Geometry check sheet. Reference: the model listing, model coordinates, mm. Coordinates: 2 decimals unless noted, no trailing zeros. Order: outer loops, then holes, each group sorted by start corner. A loop starts at its lowest first (then second) coordinate and runs counter-clockwise, first axis right, second up. Notation, with made-up numbers: (-23, -9) - (28, -9) arc R14 ccw to (28, 8) - close; hole circle Ø11 at (52.5, 81.5). An arc over 180 degrees is marked (long way). Use CSV: the item, a comma, the result in double quotes. Start each with the question number.
1) Sectioned sample at B-B, the plane z = -54. Record the cut outline in (x, y), and give its area (3 significant figures).
2) Depth check by flat-ended pin: P1, Ø1.2, axis at y = 0.5, z = -62.5, coming from the +X side; P2, Ø2.5, axis at x = 70, z = -39, coming from the -Y side; P3, Ø1.2, axis at y = 1, z = -60.5, coming from the -X side; P4, Ø1.5, axis at y = 1.5, z = -27.5, coming from the -X side. Enter the tip coordinate at first touch or a pass-through.
3) Sectioned sample at D-D, the plane y = 0.1. Count the separate pieces of the cut face and the enclosed holes in it, and give its area (3 significant figures).
4) Thickness scan on probe 1 along Z at (x, y) = (-16, -1.3); probe 2 along X at (y, z) = (0.35, -24.5); probe 3 along X at (y, z) = (0.5, -48). Record the ranges inside material, lowest first. Write a range as [from, to].
5) Sectioned sample at C-C, the plane x = 1. Record the cut outline in (y, z).
6) Sectioned sample at A-A, the plane x = 28. Record the cut outline in (y, z), and give its area (3 significant figures).
from build123d import *

# Parameters (mm, degrees)
F1_DEPTH = 2
F2_SIZE  = 5
F3_R     = 5
F4_R     = 1.5
F5_DEPTH = 4.001
F6_R     = 0.5
F8_DEPTH = 4.001


with BuildPart() as f1:
    # F0 (on Front) → F1 (new body, symmetric)
    with BuildSketch(Plane.XZ):
        with BuildLine():
            Line((94.041232037, 0), (-94.041232037, 0))
            ThreePointArc((-94.041232037, 0), (-97.8714542526, -1.7860619516), (-98.9652708021, -5.8682408883))
            Line((-98.9652708021, -5.8682408883), (-86.9750361139, -73.8682408883))
            ThreePointArc((-86.9750361139, -73.8682408883), (-85.2649353973, -76.8302222156), (-82.0509973489, -78))
            Line((-82.0509973489, -78), (-74, -78))
            Line((-74, -78), (-74, -39))
            Line((-74, -39), (-70, -39))
            Line((-70, -39), (-70, -78))
            Line((-70, -78), (70, -78))
            Line((70, -78), (70, -39))
            Line((70, -39), (74, -39))
            Line((74, -39), (74, -78))
            Line((74, -78), (82.0509973489, -78))
            ThreePointArc((82.0509973489, -78), (85.2649353973, -76.8302222156), (86.9750361139, -73.8682408883))
            Line((86.9750361139, -73.8682408883), (98.9652708021, -5.8682408883))
            ThreePointArc((98.9652708021, -5.8682408883), (97.8714542526, -1.7860619516), (94.041232037, 0))
        make_face()
    extrude(amount=F1_DEPTH, both=True)

    # F2
    f2_edges = [f1.edges().sort_by_distance(p)[0] for p in [
        (-74, 0, -78),
        (-70, 0, -78),
        (70, 0, -78),
        (74, 0, -78),
    ]]
    chamfer(f2_edges, length=F2_SIZE)

    # F3
    f3_edges = [f1.edges().sort_by_distance(p)[0] for p in [
        (74, 0, -73),
        (79, 0, -78),
        (70, 0, -73),
        (65, 0, -78),
        (-70, 0, -73),
        (-65, 0, -78),
        (-74, 0, -73),
        (-79, 0, -78),
    ]]
    fillet(f3_edges, radius=F3_R)

    # F4 (on face) → F5 (cut, through all)
    with BuildSketch(Plane.XZ.offset(2)):
        with Locations((74, -39)):
            Circle(F4_R)
        with Locations((70, -39)):
            Circle(F4_R)
        with Locations((-70, -39)):
            Circle(F4_R)
        with Locations((-74, -39)):
            Circle(F4_R)
    extrude(amount=-F5_DEPTH, mode=Mode.SUBTRACT)

    # F6
    f6_edges = [f1.edges().sort_by_distance(p)[0] for p in [
        (72.5, 0, -39),
        (74, 0, -40.5),
        (71.5, 0, -39),
        (70, 0, -40.5),
        (-74, 0, -40.5),
        (-72.5, 0, -39),
        (-71.5, 0, -39),
        (-70, 0, -40.5),
    ]]
    fillet(f6_edges, radius=F6_R)

    # F7 (on face) → F8 (cut, through all)
    with BuildSketch(Plane.XZ.offset(2)):
        with BuildLine():
            ThreePointArc((-38.884648043, -21.6798654453), (-44.0825181885, -19.2969474728), (-48.1170495204, -23.3489480955))
            Line((-48.1170495204, -23.3489480955), (-54.9555054903, -62.1317591117))
            ThreePointArc((-54.9555054903, -62.1317591117), (-53.8616889408, -66.2139380484), (-50.0314667252, -68))
            Line((-50.0314667252, -68), (-20.3526544878, -68))
            ThreePointArc((-20.3526544878, -68), (-16.0117664627, -65.4812680536), (-16.0442917755, -60.4626764615))
            Line((-16.0442917755, -60.4626764615), (-38.884648043, -21.6798654453))
        make_face()
        with BuildLine():
            ThreePointArc((-25.4106153193, -10), (-29.7515033444, -12.5187319464), (-29.7189780316, -17.5373235385))
            Line((-29.7189780316, -17.5373235385), (-4.3083627123, -60.6844216043))
            ThreePointArc((-4.3083627123, -60.6844216043), (0, -63.1470980658), (4.3083627123, -60.6844216043))
            Line((4.3083627123, -60.6844216043), (29.7189780316, -17.5373235385))
            ThreePointArc((29.7189780316, -17.5373235385), (29.7515033444, -12.5187319464), (25.4106153193, -10))
            Line((25.4106153193, -10), (-25.4106153193, -10))
        make_face()
        with BuildLine():
            ThreePointArc((50.0314667252, -68), (53.8616889408, -66.2139380484), (54.9555054903, -62.1317591117))
            Line((54.9555054903, -62.1317591117), (48.1170495204, -23.3489480955))
            ThreePointArc((48.1170495204, -23.3489480955), (44.0825181885, -19.2969474728), (38.884648043, -21.6798654453))
            Line((38.884648043, -21.6798654453), (16.0442917755, -60.4626764615))
            ThreePointArc((16.0442917755, -60.4626764615), (16.0117664627, -65.4812680536), (20.3526544878, -68))
            Line((20.3526544878, -68), (50.0314667252, -68))
        make_face()
    extrude(amount=-F8_DEPTH, mode=Mode.SUBTRACT)


solid = f1.part
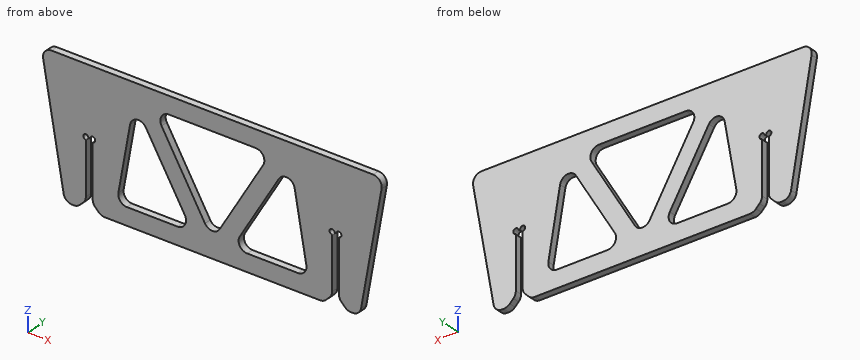
Evaluation:
1,outline,"(-90.48, -2) - (-74, -2) - (-74, 2) - (-90.48, 2) - close; (-70, -2) - (-53.52, -2) - (-53.52, 2) - (-70, 2) - close; (-19.85, -2) - (-8.25, -2) - (-8.25, 2) - (-19.85, 2) - close; (8.25, -2) - (19.85, -2) - (19.85, 2) - (8.25, 2) - close; (53.52, -2) - (70, -2) - (70, 2) - (53.52, 2) - close; (74, -2) - (90.48, -2) - (90.48, 2) - (74, 2) - close"
1,area,"356 mm²"
2,P1,"x = 89.09"
2,P2,"through"
2,P3,"x = -89.44"
2,P4,"x = -95.28"
3,separate pieces,"1"
3,enclosed holes,"3"
3,area,"9,740 mm²"
4,probe 1,"[-78, -65.46], [-60.54, -40.83], [-10, 0]"
4,probe 2,"[-95.68, -48.32], [-37.22, -25.62], [25.62, 37.22], [48.32, 95.68]"
4,probe 3,"[-91.54, -74], [-70, -52.46], [-23.38, -11.78], [11.78, 23.38], [52.46, 70], [74, 91.54]"
5,outline,"(-2, -78) - (2, -78) - (2, -63.05) - (-2, -63.05) - close; (-2, -10) - (2, -10) - (2, 0) - (-2, 0) - close"
6,outline,"(-2, -78) - (2, -78) - (2, -68) - (-2, -68) - close; (-2, -40.16) - (2, -40.16) - (2, -20.46) - (-2, -20.46) - close; (-2, -10.72) - (2, -10.72) - (2, 0) - (-2, 0) - close"
6,area,"162 mm²"
